Job drawing, mm, ordinate dimensions from the low corner. One solid piece. A direction names the side the tool comes from. Give positions to 0.01 mm unless a question says otherwise; leave off trailing zeros. Loops run counter-clockwise (first coordinate to the right, second up) from the corner with the lowest first, then second, coordinate; pieces in that order, holes last. Notation, with made-up numbers: (55.25, 84.25) - (94.25, 84.25) arc R13 cw to (94.25, 101.25) - close; hole circle Ø4 at (45.5, 38). An arc over 180 degrees is marked (long way). Answer as CSV lines item,"result". Start each with the question number.
Item 1: Pin check, flat tips, straight feed: pin 1 (5 mm diameter, centred on x = 13.5, y = 30, fed in from -Z); pin 2 (12 mm diameter, centred on x = 31, y = 7, fed in from +Z); pin 3 (1 mm diameter, centred on x = 7, z = 2, fed in from -Y); pin 4 (1 mm diameter, centred on y = 8.5, z = 1.5, fed in from +X). Stop position of each tip, or through.
Item 2: Tool access for the marked faces 1, 2 and 3: list every direction of +Z, -Z, +X, -X, +Y, -Y with a clear straight run to the whole face (end or side of a thin tool).
Item 3: Saw through at B-B on y = 16.5. Give the cut face in (x, z) (3 decimals).
Item 4: Saw through at C-C on x = 24. Give the cut face in (y, z) (3 decimals), plus the area to 3 significant figures.
Item 5: Drill centre lines: L1, parallel to Y at x = 27, z = 1.35; L2, parallel to X at y = 5.5, z = 3; L3, parallel to Y at x = 14.5, z = 0.2. Where is each one in solid material? Low to high. Write a range as from..to.
Item 6: Saw through at A-A on z = 2.45. Give the cut face in (x, y) (3 decimals), plus the area to 3 significant figures.
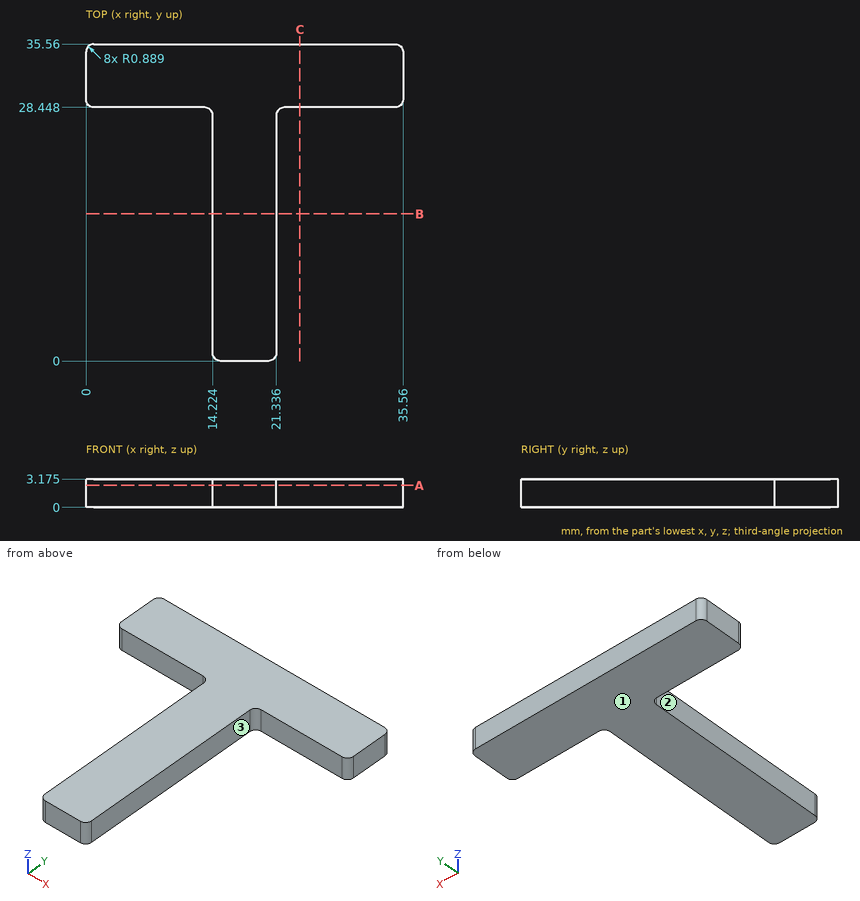
Responses:
1,pin 1,"z = 0"
1,pin 2,"through"
1,pin 3,"y = 28.45"
1,pin 4,"x = 21.34"
2,face 1,"-Z, +X, -X, +Y, -Y"
2,face 2,"+Z, -Z, -X, -Y"
2,face 3,"+Z, -Z, +X, -Y"
3,outline,"(14.224, 0) - (21.336, 0) - (21.336, 3.175) - (14.224, 3.175) - close"
4,outline,"(28.448, 0) - (35.56, 0) - (35.56, 3.175) - (28.448, 3.175) - close"
4,area,"22.6 mm2"
5,L1,"28.45..35.56"
5,L2,"14.22..21.34"
5,L3,"0.25..35.56"
6,outline,"(0, 29.337) arc R0.889 ccw to (0.889, 28.448) - (13.335, 28.448) arc R0.889 cw to (14.224, 27.559) - (14.224, 0.889) arc R0.889 ccw to (15.113, 0) - (20.447, 0) arc R0.889 ccw to (21.336, 0.889) - (21.336, 27.559) arc R0.889 cw to (22.225, 28.448) - (34.671, 28.448) arc R0.889 ccw to (35.56, 29.337) - (35.56, 34.671) arc R0.889 ccw to (34.671, 35.56) - (0.889, 35.56) arc R0.889 ccw to (0, 34.671) - close"
6,area,"455 mm2"
